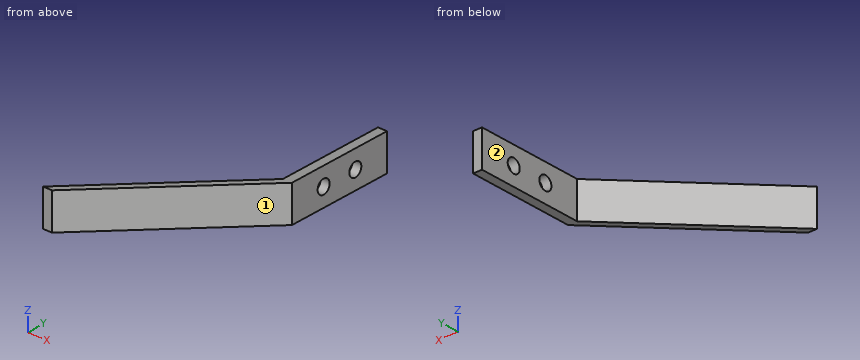
```python
from build123d import *

# Parameters (mm, degrees)
SKETCH1_W           = 6.35
SKETCH1_H           = 76.2
BOSS_EXTRUDE1_DEPTH = 25.4
SKETCH2_R           = 4.826
CUT_EXTRUDE1_DEPTH  = 25.4


with BuildPart() as part:
    # Sketch1 → Boss-Extrude1 (new body)
    with BuildSketch(Plane.XY):
        with Locations((0, 38.1)):
            Rectangle(SKETCH1_W, SKETCH1_H)
        Polygon((-92.977561211, -89.802561211), (-86.627561211, -89.802561211), (3.175, 0), (-3.175, 0), align=None)
    extrude(amount=BOSS_EXTRUDE1_DEPTH)

    # Sketch2 → Cut-Extrude1 (cut)
    with BuildSketch(Plane.ZY.offset(3.175)):
        with Locations((12.7, 50.8)):
            Circle(SKETCH2_R)
        with Locations((12.7, 25.4)):
            Circle(SKETCH2_R)
    extrude(amount=-CUT_EXTRUDE1_DEPTH, mode=Mode.SUBTRACT)


solid = part.part
```
Here's how the part is built. I have some questions about the finished solid (model axes, mm). Face numbers are marked on the shaded views. A direction names the side the tool comes from. Round coordinates to 2 decimals unless told otherwise and drop trailing zeros. Write each loop counter-clockwise with the first axis right and the second up, starting at its lowest first coordinate (ties: lowest second). Pieces come first, ordered by that corner, then holes.
Q1. If we section it at D-D on x = -42: Write out the boundary of the cut face in (y, z) (3 decimals), plus the area to 3 significant figures.
Q2. Which directions (+Z, -Z, +X, -X, +Y, -Y) give clear straight access to the entire face, cutting with the end or side of a thin tool? Please do the marked faces 1 and 2.
Q3. If we section it at A-A on z = 12.7: Write out the boundary of the cut face in (x, y) (3 decimals).
Q4. Will these pins go through, and if not, where does the flat tip stop? P1, Ø12, axis at y = -30.5, z = 10, coming from the -X side (3 decimals); P2, Ø8, axis at y = -7, z = 6, coming from the -X side (3 decimals); P3, Ø6, axis at x = -48, z = 6, coming from the +Y side (3 decimals).
Q5. Please list where these lines run through material, in increasing order: probe 1 along Y at (x, z) = (-0.25, 12.7) (3 decimals); probe 2 along Y at (x, z) = (2, 12.7) (3 decimals); probe 3 along X at (y, z) = (17.5, 18) (3 decimals).
Q6. If we section it at B-B on y = 50.8: Write out the boundary of the cut face in (x, z) (3 decimals), plus the area to 4 significant figures.
Q7. If we section it at C-C on z = 3: Write out the boundary of the cut face in (x, y) (3 decimals).
Answer below:
1. outline: (-45.175, 0) - (-38.825, 0) - (-38.825, 25.4) - (-45.175, 25.4) - close
1. area: 161 mm2
2. face 1: +Z, -Z, +X, -Y
2. face 2: +Z, -Z, -X, +Y
3. outline: (-92.978, -89.803) - (-86.628, -89.803) - (3.175, 0) - (3.175, 20.574) - (-3.175, 20.574) - (-3.175, 0) - close; (-3.175, 30.226) - (3.175, 30.226) - (3.175, 45.974) - (-3.175, 45.974) - close; (-3.175, 55.626) - (3.175, 55.626) - (3.175, 76.2) - (-3.175, 76.2) - close
4. P1: stops at x = -39.675
4. P2: stops at x = -14.175
4. P3: stops at y = -41.825
5. probe 1: y = -3.425 to 20.574, 30.226 to 45.974, 55.626 to 76.2
5. probe 2: y = -1.175 to 20.574, 30.226 to 45.974, 55.626 to 76.2
5. probe 3: x = -3.175 to 3.175
6. outline: (-3.175, 0) - (3.175, 0) - (3.175, 7.874) - (-3.175, 7.874) - close; (-3.175, 17.526) - (3.175, 17.526) - (3.175, 25.4) - (-3.175, 25.4) - close
6. area: 100.0 mm2
7. outline: (-92.978, -89.803) - (-86.628, -89.803) - (3.175, 0) - (3.175, 76.2) - (-3.175, 76.2) - (-3.175, 0) - close
